Verification items for this drawing (mm, ordinates from the low corner). A direction names the side the tool comes from. Give positions to 0.01 mm unless a question says otherwise; leave off trailing zeros. Loops run counter-clockwise (first coordinate to the right, second up) from the corner with the lowest first, then second, coordinate; pieces in that order, holes last. Notation, with made-up numbers: (30, 11) -> (52, 11) arc R22 ccw to (52, 33) -> close; hole circle Ø11 at (28, -30). An arc over 180 degrees is marked (long way). Write each question's results on one line, items separated by ' | '. Start each with the question number.
1) Sectioned sample at B-B on z = 39.5. Record the cut outline in (x, y), then the cut area to 3 significant figures.
2) Depth check by flat-ended pin: pin 1 (12 mm diameter, centred on y = 15.5, z = 38.5, fed in from +X); pin 2 (1.5 mm diameter, centred on y = 7, z = 37.5, fed in from +X) (3 decimals); pin 3 (4 mm diameter, centred on y = 34.5, z = 24.5, fed in from +X). Enter the tip coordinate at first touch or a pass-through.
3) Sectioned sample at D-D on x = 67.5. Record the cut outline in (y, z).
4) Scan lines: line 1 (Y direction, x = 6, z = 5.5); line 2 (Z direction, x = 75, y = 21); line 3 (Z direction, x = 74, y = 50). Record each from-to range of solid material in increasing order. Write a range as from..to.
5) Sectioned sample at C-C on y = 34. Record the cut outline in (x, z), then the cut area to 3 significant figures.
6) Sectioned sample at A-A on x = 15.5. Record the cut outline in (y, z), then the cut area to 3 significant figures.
7) Draft check along Y on the marked faces 1, 2, 3 and 4. Enter one of: pulls with the +Y half, pulls with the -Y half, needs draft (parallel to the pull), parting line crosses it, or undercut.
8) Set-up check for the marked faces 5, 6 and 7: record each of +Z, -Z, +X, -X, +Y, -Y from which the full face is reachable in a straight line by a thin tool's end or side.
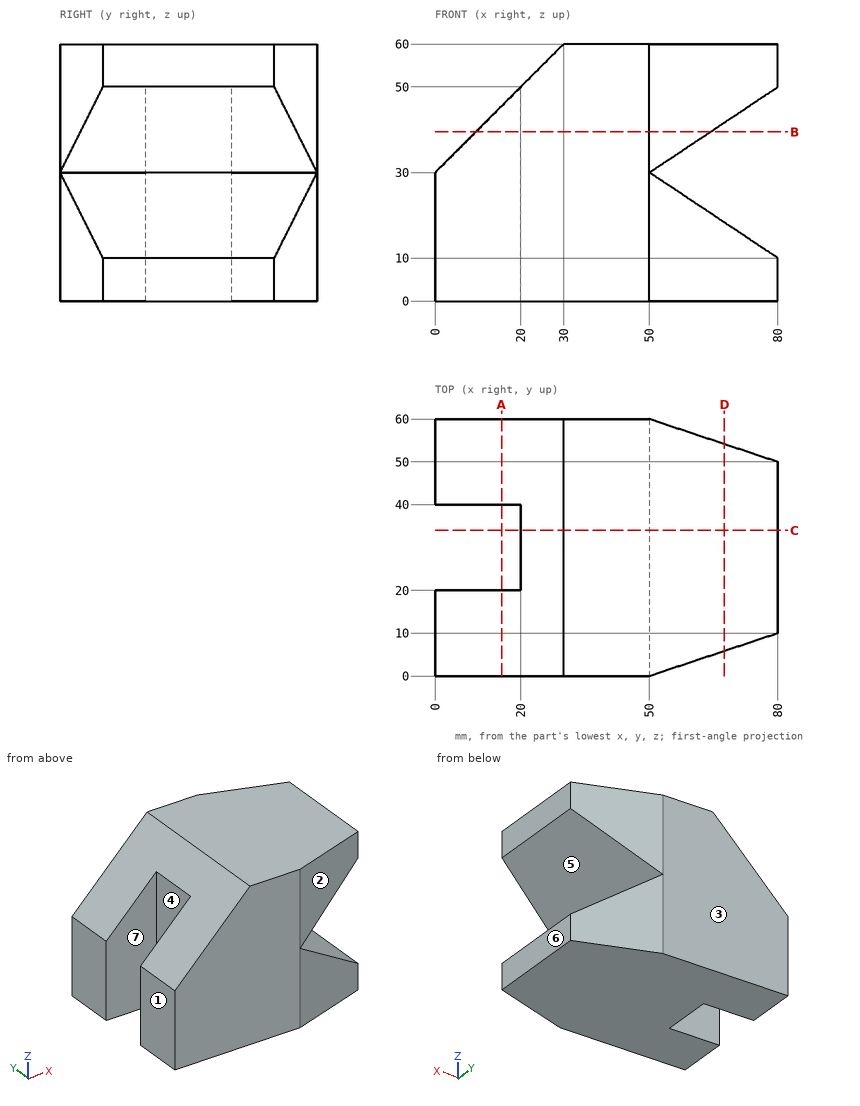
Result:
1) outline: (9.5, 0) -> (50, 0) -> (64.25, 4.75) -> (64.25, 55.25) -> (50, 60) -> (9.5, 60) -> (9.5, 40) -> (20, 40) -> (20, 20) -> (9.5, 20) -> close | area: 3,010 mm^2
2) pin 1: x = 71.75 | pin 2: x = 62.375 | pin 3: x = 61.25
3) outline: (5.83, 0) -> (54.17, 0) -> (54.17, 18.33) -> (5.83, 18.33) -> close; (5.83, 41.67) -> (54.17, 41.67) -> (54.17, 60) -> (5.83, 60) -> close
4) line 1: 0..20, 40..60 | line 2: 0..13.33, 46.67..60 | line 3: 0..14, 46..60
5) outline: (20, 0) -> (80, 0) -> (80, 10) -> (50, 30) -> (80, 50) -> (80, 60) -> (30, 60) -> (20, 50) -> close | area: 2,950 mm^2
6) outline: (0, 0) -> (20, 0) -> (20, 45.5) -> (0, 45.5) -> close; (40, 0) -> (60, 0) -> (60, 45.5) -> (40, 45.5) -> close | area: 1,820 mm^2
7) face 1: needs draft | face 2: pulls with the -Y half | face 3: pulls with the +Y half | face 4: undercut
8) face 5: +X, +Y, -Y | face 6: +Z, -Z, +X, +Y, -Y | face 7: +Z, -Z, -X
